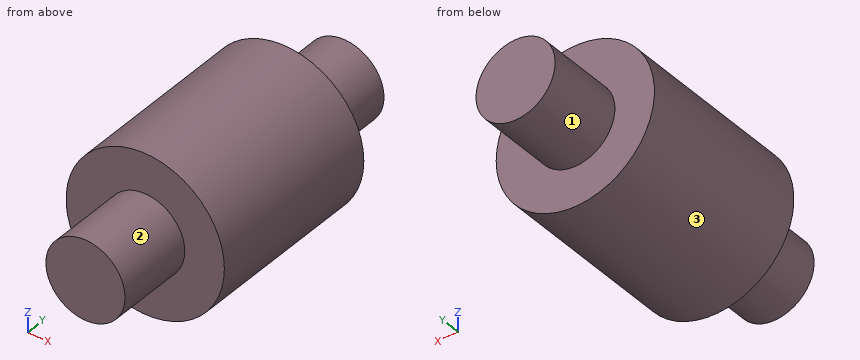
```python
from build123d import *

# Parameters (mm, degrees)
SKETCH_1_R      = 3
EXTRUDE_1_DEPTH = 7
SKETCH_2_R      = 1.5
EXTRUDE_2_DEPTH = 3
SKETCH_3_R      = 1.5
EXTRUDE_3_DEPTH = 3


with BuildPart() as part:
    # Эскиз1 → Бобышка-Вытянуть1 (new body)
    with BuildSketch(Plane(origin=(0, 0, 0), x_dir=(1, 0, 0), z_dir=(0, 1, 0))):
        Circle(SKETCH_1_R)
    extrude(amount=EXTRUDE_1_DEPTH)

    # Эскиз2 → Бобышка-Вытянуть2 (add)
    with BuildSketch(Plane.XZ):
        Circle(SKETCH_2_R)
    extrude(amount=EXTRUDE_2_DEPTH)

    # Эскиз3 → Бобышка-Вытянуть3 (add)
    with BuildSketch(Plane(origin=(0, 7, 0), x_dir=(1, 0, 0), z_dir=(0, 1, 0))):
        Circle(SKETCH_3_R)
    extrude(amount=EXTRUDE_3_DEPTH)


solid = part.part
```
Work out the finished part from the listing and answer in its coordinate system (mm). Face numbers are marked on the shaded views. A direction names the side the tool comes from. Coordinates: 2 decimals unless noted, no trailing zeros. Write each loop counter-clockwise with the first axis right and the second up, starting at its lowest first coordinate (ties: lowest second). Pieces come first, ordered by that corner, then holes.
Q1. A cutting plane is placed at C-C, the plane y = 2.5. Give the vertices of the cut face in (x, z).
Q2. A cutting plane is placed at D-D, the plane z = -1.65. Give the vertices of the cut face in (x, y), then the cut area to 3 significant figures.
Q3. A cutting plane is placed at B-B, the plane x = 0. Give the vertices of the cut face in (y, z).
Q4. A cutting plane is placed at A-A, the plane z = 0. Give the vertices of the cut face in (x, y).
Q5. Each of these flat-tipped pins is pushed along its axis until it touches: pin 1 Ø1 at (y, z) = (2, 1) entering from +X; pin 2 Ø1.5 at (y, z) = (8.5, 0) entering from +X. Where does it stop, or does it pass through?
Q6. Which of the six approach directions +Z, -Z, +X, -X, +Y, -Y give full straight-line access (tool end or side, diameter ignored) to the marked faces 1, 2 and 3?
Q7. Find the intervals of material crossed by line 1 (Y direction, x = 1, z = 1.65); line 2 (Z direction, x = 0.15, y = 5.5); line 3 (X direction, y = 4.5, z = 2.6), in increasing order.
Findings below:
1. outline: circle Ø6 at (0, 0)
2. outline: (-2.51, 0) - (2.51, 0) - (2.51, 7) - (-2.51, 7) - close
2. area: 35.1 mm2
3. outline: (-3, -1.5) - (0, -1.5) - (0, -3) - (7, -3) - (7, -1.5) - (10, -1.5) - (10, 1.5) - (7, 1.5) - (7, 3) - (0, 3) - (0, 1.5) - (-3, 1.5) - close
4. outline: (-3, 0) - (-1.5, 0) - (-1.5, -3) - (1.5, -3) - (1.5, 0) - (3, 0) - (3, 7) - (1.5, 7) - (1.5, 10) - (-1.5, 10) - (-1.5, 7) - (-3, 7) - close
5. pin 1: stops at x = 2.96
5. pin 2: stops at x = 1.5
6. face 1: +Y
6. face 2: -Y
6. face 3: +Y, -Y
7. line 1: y = 0 to 7
7. line 2: z = -3 to 3
7. line 3: x = -1.5 to 1.5
